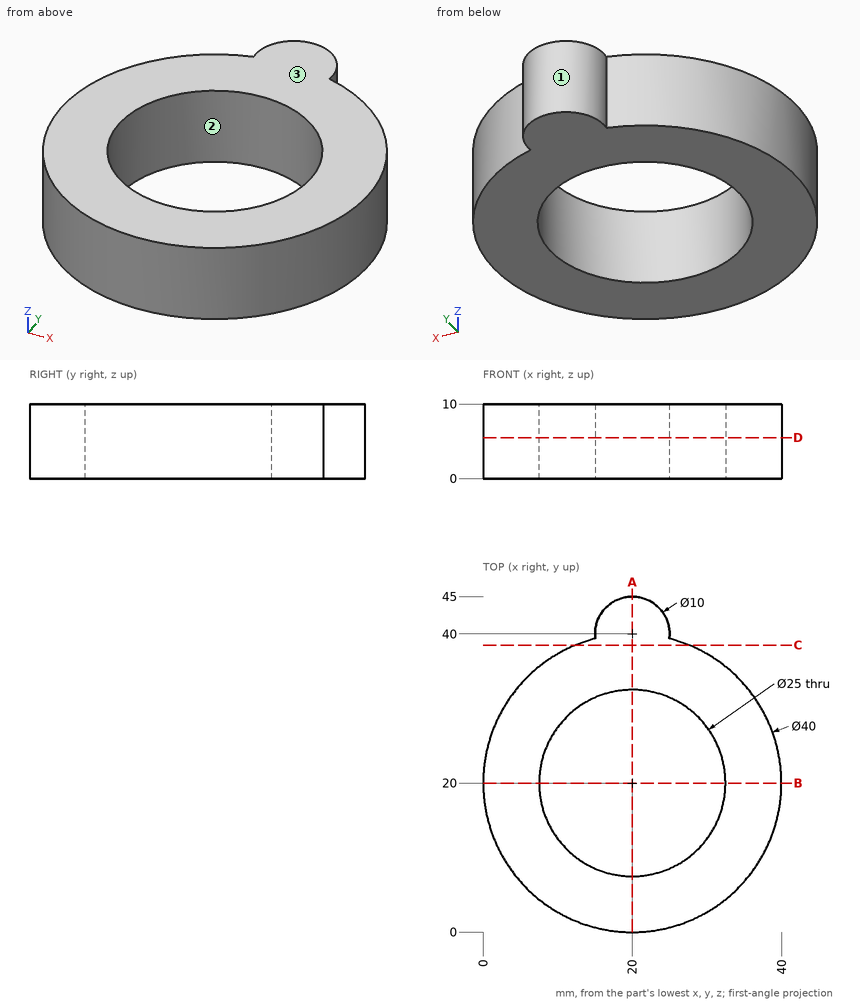
Job drawing, mm, ordinate dimensions from the low corner. One solid piece. Coordinates: 2 decimals unless noted, no trailing zeros. Write each loop counter-clockwise with the first axis right and the second up, starting at its lowest first coordinate (ties: lowest second). Pieces come first, ordered by that corner, then holes. Notation, with made-up numbers: M 56.5,78.25 L 80.5,78.25 A18 ccw 80.5,84.25 Z; hole C -32,48.5 d2. An arc over 180 degrees is marked long. Answer as a JSON object with one key per item and string values. Group by question number.
1) Pin check, flat tips, straight feed: pin 1 Ø3 at (x, z) = (8, 4) entering from -Y; pin 2 Ø2 at (x, z) = (33, 3.5) entering from -Y; pin 3 Ø1.5 at (x, z) = (15, 4.5) entering from +Y. Stop position of each tip, or through.
2) Saw through at B-B (y = 20). Write the cut outline in (x, z).
3) Saw through at A-A (x = 20). Write the cut outline in (y, z), plus the area to 3 significant figures.
4) Saw through at C-C (y = 38.5). Write the cut outline in (x, z), plus the area to 3 significant figures.
5) Wall check: line 1 (X direction, y = 19.5, z = 6.75); line 2 (X direction, y = 9.5, z = 3.25); line 3 (Y direction, x = 12, z = 9). Give the ranges that are in metal, low to high. Write a range as from..to.
6) Saw through at D-D (z = 5.5). Write the cut outline in (x, y) (3 decimals), plus the area to 3 significant figures.
7) Mould opens along X. For the marked faces 1, 2 and 3 say: +X half, -X half, draft (parallel to the pull), parting line (faces both ways), or undercut.
Values follow:
{
 "1": {"pin 1": "stops at y = 2.98", "pin 2": "stops at y = 4", "pin 3": "stops at y = 42.63"},
 "2": {"outline": "M 0,0 L 7.5,0 L 7.5,10 L 0,10 Z; M 32.5,0 L 40,0 L 40,10 L 32.5,10 Z"},
 "3": {"outline": "M 0,0 L 7.5,0 L 7.5,10 L 0,10 Z; M 32.5,0 L 45,0 L 45,10 L 32.5,10 Z", "area": "200 mm2"},
 "4": {"outline": "M 12.4,0 L 27.6,0 L 27.6,10 L 12.4,10 Z", "area": "152 mm2"},
 "5": {"line 1": "x = 0.01..7.51, 32.49..39.99", "line 2": "x = 2.98..13.22, 26.78..37.02", "line 3": "y = 1.67..10.4, 29.6..38.33"},
 "6": {"outline": "M 15.039,39.375 A20 ccw long 24.961,39.375 A5 ccw long Z; hole C 20,20 d25", "area": "807 mm2"},
 "7": {"face 1": "parting line", "face 2": "undercut", "face 3": "draft"}
}
